Geometry check sheet. Reference: the model listing, model coordinates, mm. Face numbers are marked on the shaded views. A direction names the side the tool comes from. Give positions to 0.01 mm unless a question says otherwise; leave off trailing zeros. Order: outer loops, then holes, each group sorted by start corner. A loop starts at its lowest first (then second) coordinate and runs counter-clockwise, first axis right, second up. Notation, with made-up numbers: M 14,10 L 57,10 A27 ccw 57,38 Z; hole C -6.75,39.5 d6. An arc over 180 degrees is marked long. Answer as CSV lines item,"result". Start each with the question number.
Q1. Section check C-C, the plane z = 33. Count the separate pieces of the cut face and the enclosed holes in it, then the cut area to 3 significant figures.
Q2. Mould release check, pull along X, two halves, no side actions. Record for the marked faces 1, 2, 3 and 4: +X half, -X half, draft (parallel to the pull), parting line (faces both ways), or undercut.
Q3. Section check A-A, the plane x = 20.64. Record the boundary of the cut face in (y, z), then the cut area to 3 significant figures.
Q4. Set-up check for the marked faces 5, 6 and 7: record each of +Z, -Z, +X, -X, +Y, -Y from which the full face is reachable in a straight line by a thin tool's end or side.
Q5. Go/stop test with flat-tipped pins: pin 1 (7 mm diameter, centred on y = 16.5, z = -23, fed in from +X); pin 2 (6.5 mm diameter, centred on x = -20.64, z = 31.75, fed in from +Y); pin 3 (10.5 mm diameter, centred on y = 24, z = -7, fed in from -X). Record where each tip stops, or that it passes through.
Q6. Thickness scan on line 1 (X direction, y = 3.75, z = -31.75); line 2 (Z direction, x = 20.64, y = 1.6); line 3 (Z direction, x = 20, y = 3). Record the ranges inside material, lowest first.
Q7. Section check B-B, the plane x = 11. Record the boundary of the cut face in (y, z), then the cut area to 3 significant figures.
```python
from build123d import *
from OCP.BRepFilletAPI import BRepFilletAPI_MakeChamfer

# Parameters (mm, degrees)
SKETCH1_W                  = 55
SKETCH1_H                  = 77
BOSS_EXTRUDE1_DEPTH        = 45
CUT_EXTRUDE1_DEPTH         = 66.295482233
CUT_EXTRUDE1_DEPTH_BACK    = 66.295482233
SKETCH2_W                  = 15
SKETCH2_H                  = 45
CUT_EXTRUDE2_DEPTH         = 61.526853545
CUT_EXTRUDE2_DEPTH_BACK    = 61.526853545
SKETCH9_R                  = 4.7625
CUT_EXTRUDE5_DEPTH         = 60.605373357
CUT_EXTRUDE4_DEPTH         = 7.5
CUT_EXTRUDE4_DEPTH_BACK    = 7.5
CHAMFER1_SIZE              = 5
FILLET1_R                  = 4
F_12_0MM_DOWEL_HOLE2_D     = 18
F_12_0MM_DOWEL_HOLE2_DEPTH = 12
F_12_0MM_DOWEL_HOLE2_TIP   = 5.407745571
CUT_EXTRUDE6_DEPTH         = 59.947948642
CUT_EXTRUDE6_DEPTH_BACK    = 59.947948642
SKETCH16_W                 = 77
SKETCH16_H                 = 0.28
SKETCH17_W                 = 15
SKETCH17_H                 = 77
BOSS_EXTRUDE2_DEPTH        = 5
SKETCH18_R                 = 2.75
CUT_EXTRUDE8_DEPTH         = 10
FILLET2_R                  = 4
CHAMFER2_SIZE              = 0.5
CHAMFER2_SIZE2             = 4.056570221


with BuildPart() as part:
    # Sketch1 → Boss-Extrude1 (new body)
    with BuildSketch(Plane(origin=(0, 0, 0), x_dir=(1, 0, 0), z_dir=(0, 1, 0))):
        Rectangle(SKETCH1_W, SKETCH1_H)
    extrude(amount=BOSS_EXTRUDE1_DEPTH)

    # Sketch2 → Cut-Extrude1 (cut, two sides: drawn at the far end of the back side and taken through both)
    with BuildSketch(Plane.XY.offset(-CUT_EXTRUDE1_DEPTH_BACK)):
        with Locations((-20, 22.5)):
            Rectangle(SKETCH2_W, SKETCH2_H)
        with Locations((20, 22.5)):
            Rectangle(SKETCH2_W, SKETCH2_H)
    extrude(amount=CUT_EXTRUDE1_DEPTH + CUT_EXTRUDE1_DEPTH_BACK, mode=Mode.SUBTRACT)

    # Sketch3 → Cut-Extrude2 (cut, two sides: drawn at the far end of the back side and taken through both)
    with BuildSketch(Plane(origin=(0, 0, 0), x_dir=(0, 0, -1), z_dir=(1, 0, 0)).offset(-CUT_EXTRUDE2_DEPTH_BACK)):
        Polygon((-38.5, 15), (-31.51055999, 23.329690242), (-30.745642734, 24.241283129), (-10.508137558, 7.26), (-0.650260841, 7.26), (-0.650260841, 10.26), (26.698327812, 42.85277878), (38.5, 32.95), (38.5, 45), (24.14, 45), (-38.5, 45), align=None)
    extrude(amount=CUT_EXTRUDE2_DEPTH + CUT_EXTRUDE2_DEPTH_BACK, mode=Mode.SUBTRACT)

    # Sketch9 → Cut-Extrude5 (cut, through all)
    with BuildSketch(Plane(origin=(0, 4.559375807, 5.433652498), x_dir=(1, 0, 0), z_dir=(0, 0.6427876096865435, 0.7660444431189747))):
        with Locations(Location((0, 38.806982034, 0), (0, 0, 270))):
            Circle(SKETCH9_R)
    extrude(amount=-CUT_EXTRUDE5_DEPTH, mode=Mode.SUBTRACT)

    # Sketch5 → Cut-Extrude4 (cut, two sides: drawn at the far end of the back side and taken through both)
    with BuildSketch(Plane(origin=(0, 0, 0), x_dir=(0, 0, -1), z_dir=(1, 0, 0)).offset(-CUT_EXTRUDE4_DEPTH_BACK)):
        Polygon((38.5, 0), (38.5, 30), (13.327011065, 0), align=None)
    extrude(amount=CUT_EXTRUDE4_DEPTH + CUT_EXTRUDE4_DEPTH_BACK, mode=Mode.SUBTRACT)

    # Chamfer1
    chamfer1_edges = [part.edges().sort_by_distance(p)[0] for p in [
        (-12.5, 19.620641565, 34.622821367),
        (-12.5, 37.90138939, -32.599163906),
        (12.5, 19.620641565, 34.622821367),
        (12.5, 37.90138939, -32.599163906),
    ]]
    chamfer(chamfer1_edges, length=CHAMFER1_SIZE)

    # Fillet1
    fillet1_edges = [part.edges().sort_by_distance(p)[0] for p in [
        (0, 10.26, 0.650260841),
        (0, 7.26, 10.508137558),
    ]]
    fillet(fillet1_edges, radius=FILLET1_R)

    # Ø12.0mm Dowel Hole2
    with Locations(Plane(origin=(0, -0.913904784, 0.766857167), x_dir=(1, 0, 0), z_dir=(0, 0.7660444431189749, -0.6427876096865432))):
        with Locations((0, -25.333129579)):
            Hole(F_12_0MM_DOWEL_HOLE2_D / 2, depth=F_12_0MM_DOWEL_HOLE2_DEPTH)
            with Locations((0, 0, -(F_12_0MM_DOWEL_HOLE2_DEPTH + F_12_0MM_DOWEL_HOLE2_TIP / 2))):  # 118° drill point
                Cone(0, F_12_0MM_DOWEL_HOLE2_D / 2, F_12_0MM_DOWEL_HOLE2_TIP, mode=Mode.SUBTRACT)

    # Sketch16 → Cut-Extrude6 (cut, two sides: drawn at the far end of the back side and taken through both)
    with BuildSketch(Plane(origin=(0, 0, 0), x_dir=(0, 0, -1), z_dir=(1, 0, 0)).offset(-CUT_EXTRUDE6_DEPTH_BACK)):
        with Locations((0, 0.14)):
            Rectangle(SKETCH16_W, SKETCH16_H)
    extrude(amount=CUT_EXTRUDE6_DEPTH + CUT_EXTRUDE6_DEPTH_BACK, mode=Mode.SUBTRACT)

    # Sketch17 → Boss-Extrude2 (add)
    with BuildSketch(Plane.XZ.offset(-0.28)):
        with Locations((-20, 0)):
            Rectangle(SKETCH17_W, SKETCH17_H)
        with Locations((20, 0)):
            Rectangle(SKETCH17_W, SKETCH17_H)
    extrude(amount=-BOSS_EXTRUDE2_DEPTH)

    # Sketch18 → Cut-Extrude8 (cut)
    with BuildSketch(Plane(origin=(0, 0, 0), x_dir=(1, 0, 0), z_dir=(0, 1, 0))):
        with Locations(Location((-20.64, -31.75, 0), (0, 0, 270))):
            Circle(SKETCH18_R)
        with Locations(Location((-20.64, 31.75, 0), (0, 0, 270))):
            Circle(SKETCH18_R)
        with Locations(Location((-20.64, -22.23, 0), (0, 0, 270))):
            Circle(SKETCH18_R)
        with Locations(Location((20.64, -22.23, 0), (0, 0, 270))):
            Circle(SKETCH18_R)
        with Locations(Location((20.64, 31.75, 0), (0, 0, 270))):
            Circle(SKETCH18_R)
        with Locations(Location((20.64, -31.75, 0), (0, 0, 270))):
            Circle(SKETCH18_R)
    extrude(amount=CUT_EXTRUDE8_DEPTH, mode=Mode.SUBTRACT)

    # Fillet2
    fillet2_edges = [part.edges().sort_by_distance(p)[0] for p in [
        (27.5, 2.78, -38.5),
        (27.5, 2.78, 38.5),
        (-27.5, 2.78, -38.5),
        (-27.5, 2.78, 38.5),
    ]]
    fillet(fillet2_edges, radius=FILLET2_R)

    # Chamfer2: one chamfer whose edges measure the first distance from different faces: ONE call of the kernel's chamfer builder (chamfer() names one face for all edges)
    chamfer2_edges_1 = [part.edges().sort_by_distance(p)[0] for p in [
        (-7.5, 15.14, -38.5),
        (-7.5, 0.28, -26.030979481),
        (7.5, 0.28, -26.030979481),
        (7.5, 15.14, -38.5),
        (-18, 5.28, -38.5),
        (-26.328427125, 5.28, -37.328427125),
        (-27.5, 5.28, 0),
        (-26.328427125, 5.28, 37.328427125),
        (-18, 5.28, 38.5),
        (18, 5.28, -38.5),
        (26.328427125, 5.28, -37.328427125),
        (27.5, 5.28, 0),
        (26.328427125, 5.28, 37.328427125),
        (18, 5.28, 38.5),
    ]]
    chamfer2_edges_2 = [part.edges().sort_by_distance(p)[0] for p in [
        (0, 0.28, -13.561958961),
    ]]
    chamfer2_side_2 = [part.faces().sort_by_distance(p)[0] for p in [
        (0, 14.020211625, -25.091365468),
    ]]
    chamfer2 = BRepFilletAPI_MakeChamfer(part.part.solid().wrapped)
    for e in chamfer2_edges_1:
        chamfer2.Add(CHAMFER2_SIZE, e.wrapped)
    for e in chamfer2_edges_2:
        chamfer2.Add(CHAMFER2_SIZE, CHAMFER2_SIZE2, e.wrapped, chamfer2_side_2[0].wrapped)  # the first distance lies on this face
    add(Compound.cast(chamfer2.Shape()), mode=Mode.REPLACE)


solid = part.part
```
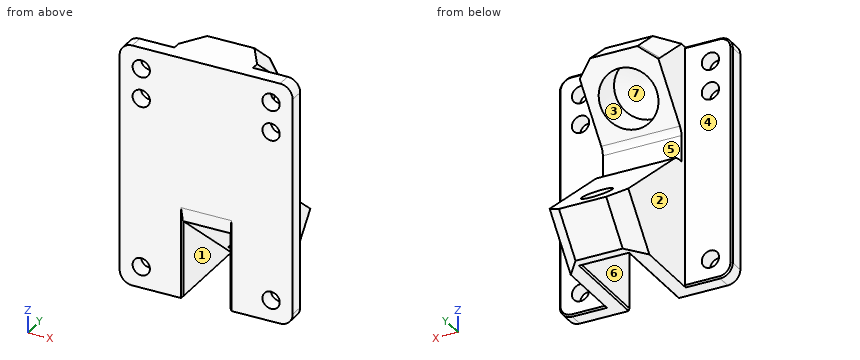
Answer block:
1,separate pieces,"3"
1,enclosed holes,"1"
1,area,"537 mm2"
2,face 1,"undercut"
2,face 2,"-X half"
2,face 3,"undercut"
2,face 4,"draft"
3,outline,"M 0.28,-38.5 L 4.78,-38.5 L 5.28,-38 L 5.28,-34.5 L 0.28,-34.5 Z; M 0.28,-29 L 5.28,-29 L 5.28,19.48 L 0.28,19.48 Z; M 0.28,24.98 L 5.28,24.98 L 5.28,29 L 0.28,29 Z; M 0.28,34.5 L 5.28,34.5 L 5.28,38 L 4.78,38.5 L 0.28,38.5 Z"
3,area,"302 mm2"
4,face 5,"+X, -X, +Y"
4,face 6,"-Z, -Y"
4,face 7,"none"
5,pin 1,"stops at x = 12.5"
5,pin 2,"stops at y = 5.28"
5,pin 3,"stops at x = -12.5"
6,line 1,"x = -27.5 to -23.39, -17.89 to -7.5, 7.5 to 17.89, 23.39 to 27.5"
6,line 2,"z = -38.5 to -34.5, -29 to 19.48, 24.98 to 29, 34.5 to 38.5"
6,line 3,"z = -38.5 to -34.42, -29.08 to 19.56, 24.9 to 29.08, 34.42 to 38.5"
7,outline,"M 0.28,-38.5 L 28.38,-38.5 L 40.17,-24.45 L 11.38,-0.29 A4 ccw 8.8,0.65 L 7.26,0.65 L 7.26,9.05 A4 cw 8.2,11.62 L 21.99,28.06 L 9.55,38.5 L 0.28,38.5 Z"
7,area,"1,590 mm2"
